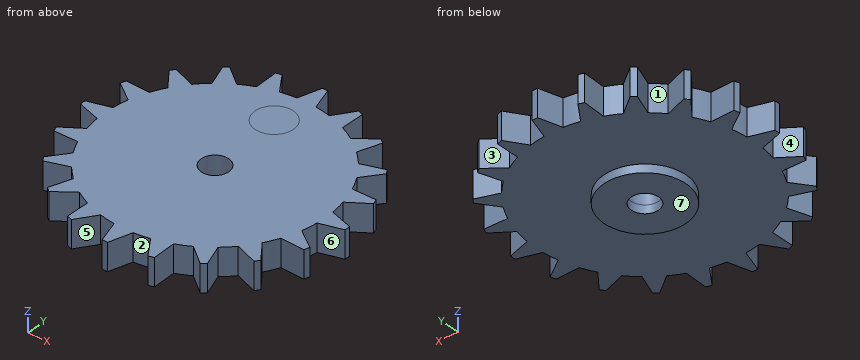
from build123d import *

# Parameters (mm, degrees)
SKETCH1_R           = 40
BOSS_EXTRUDE1_DEPTH = 10
SKETCH2_R           = 5
CUT_EXTRUDE1_DEPTH  = 10
BOSS_EXTRUDE2_DEPTH = 10
SKETCH4_R           = 5
BOSS_EXTRUDE3_DEPTH = 0.0001
SKETCH5_R           = 7
BOSS_EXTRUDE4_DEPTH = 0.0001
SKETCH6_R           = 15
BOSS_EXTRUDE5_DEPTH = 3
CUT_EXTRUDE2_START  = -3
SKETCH7_R           = 5
CUT_EXTRUDE2_DEPTH  = 3


with BuildPart() as part:
    # Sketch1 → Boss-Extrude1 (new body)
    with BuildSketch(Plane.XY):
        Circle(SKETCH1_R)
    extrude(amount=BOSS_EXTRUDE1_DEPTH)

    # Sketch2 → Cut-Extrude1 (cut)
    with BuildSketch(Plane.XY.offset(10)):
        Circle(SKETCH2_R)
    extrude(amount=-CUT_EXTRUDE1_DEPTH, mode=Mode.SUBTRACT)

    # Sketch3 → Boss-Extrude2 (add)
    with BuildSketch(Plane.XY.offset(10)):
        Polygon((-1, 48), (1, 48), (4, 38), (-4, 38), align=None)
        Polygon((7.938419721, 37.376215597), (13.881759214, 45.959729777), (15.783872246, 45.341695788), (15.546871851, 34.904079642), align=None)
        Polygon((19.09977161, 33.093786795), (27.404675116, 39.420600982), (29.022709104, 38.245030478), (25.571907565, 28.391504777), align=None)
        Polygon((28.391504777, 25.571907565), (38.245030478, 29.022709104), (39.420600982, 27.404675116), (33.093786795, 19.09977161), align=None)
        Polygon((34.904079642, 15.546871851), (45.341695788, 15.783872246), (45.959729777, 13.881759214), (37.376215597, 7.938419721), align=None)
        Polygon((38, 4), (48, 1), (48, -1), (38, -4), align=None)
        Polygon((37.376215597, -7.938419721), (45.959729777, -13.881759214), (45.341695788, -15.783872246), (34.904079642, -15.546871851), align=None)
        Polygon((33.093786795, -19.09977161), (39.420600982, -27.404675116), (38.245030478, -29.022709104), (28.391504777, -25.571907565), align=None)
        Polygon((25.571907565, -28.391504777), (29.022709104, -38.245030478), (27.404675116, -39.420600982), (19.09977161, -33.093786795), align=None)
        Polygon((15.546871851, -34.904079642), (15.783872246, -45.341695788), (13.881759214, -45.959729777), (7.938419721, -37.376215597), align=None)
        Polygon((4, -38), (1, -48), (-1, -48), (-4, -38), align=None)
        Polygon((-7.938419721, -37.376215597), (-13.881759214, -45.959729777), (-15.783872246, -45.341695788), (-15.546871851, -34.904079642), align=None)
        Polygon((-19.09977161, -33.093786795), (-27.404675116, -39.420600982), (-29.022709104, -38.245030478), (-25.571907565, -28.391504777), align=None)
        Polygon((-28.391504777, -25.571907565), (-38.245030478, -29.022709104), (-39.420600982, -27.404675116), (-33.093786795, -19.09977161), align=None)
        Polygon((-34.904079642, -15.546871851), (-45.341695788, -15.783872246), (-45.959729777, -13.881759214), (-37.376215597, -7.938419721), align=None)
        Polygon((-38, -4), (-48, -1), (-48, 1), (-38, 4), align=None)
        Polygon((-37.376215597, 7.938419721), (-45.959729777, 13.881759214), (-45.341695788, 15.783872246), (-34.904079642, 15.546871851), align=None)
        Polygon((-33.093786795, 19.09977161), (-39.420600982, 27.404675116), (-38.245030478, 29.022709104), (-28.391504777, 25.571907565), align=None)
        Polygon((-25.571907565, 28.391504777), (-29.022709104, 38.245030478), (-27.404675116, 39.420600982), (-19.09977161, 33.093786795), align=None)
        Polygon((-15.546871851, 34.904079642), (-15.783872246, 45.341695788), (-13.881759214, 45.959729777), (-7.938419721, 37.376215597), align=None)
    extrude(amount=-BOSS_EXTRUDE2_DEPTH)

    # Sketch4 → Boss-Extrude3 (add)
    with BuildSketch(Plane.XY.offset(10)):
        with Locations((-1.366858005, 27.473845905)):
            Circle(SKETCH4_R)
    extrude(amount=BOSS_EXTRUDE3_DEPTH)

    # Sketch5 → Boss-Extrude4 (add)
    with BuildSketch(Plane.XY.offset(10)):
        with Locations((-1.366858005, 27.473845905)):
            Circle(SKETCH5_R)
    extrude(amount=BOSS_EXTRUDE4_DEPTH)

    # Sketch6 → Boss-Extrude5 (add)
    with BuildSketch(Plane(origin=(0, 0, 0), x_dir=(-1, 0, 0), z_dir=(0, 0, -1))):
        with Locations(Location((0, 0, 0), (0, 0, 180))):
            Circle(SKETCH6_R)
    extrude(amount=BOSS_EXTRUDE5_DEPTH)

    # Sketch7 → Cut-Extrude2 (cut)
    with BuildSketch(Plane(origin=(0, 0, -3), x_dir=(-1, 0, 0), z_dir=(0, 0, -1)).offset(CUT_EXTRUDE2_START)):
        with Locations(Location((0, 0, 0), (0, 0, 180))):
            Circle(SKETCH7_R)
    extrude(amount=CUT_EXTRUDE2_DEPTH, mode=Mode.SUBTRACT)


solid = part.part
Source: CAD feature listing. Evaluate the final solid. Frame: model axes, mm. Face numbers are marked on the shaded views. A direction names the side the tool comes from. Round coordinates to 2 decimals unless told otherwise and drop trailing zeros. Order: outer loops, then holes, each group sorted by start corner. A loop starts at its lowest first (then second) coordinate and runs counter-clockwise, first axis right, second up. Notation, with made-up numbers: (38, -14) - (87, -14) arc R21 ccw to (87, -6) - close; hole circle Ø9 at (19, 53.5). An arc over 180 degrees is marked (long way). Use a Markdown table: item, result. Add a question column.
1. Section query A-A (y = -32). Return the cut outline in (x, z).
2. First-contact query: pin 1 (1 mm diameter, centred on y = 31.5, z = 8, fed in from -X); pin 2 (1 mm diameter, centred on x = -21.5, z = 8.5, fed in from +Y); pin 3 (6 mm diameter, centred on x = 32.5, y = 17.5, fed in from -Z); pin 4 (11.5 mm diameter, centred on x = 0, y = 0, fed in from -Z). Flat tips, straight axial feed; report the tip coordinate or a pass-through.
3. Set-up query: the marked faces 1, 2, 3 and 4. Return all of +Z, -Z, +X, -X, +Y, -Y with unobstructed straight access to the full face (end or side cutting, diameter ignored); none if empty.
4. Line query: probe 1 along Y at (x, z) = (0, -1.1); probe 2 along Y at (x, z) = (0, 3.75); probe 3 along X at (y, z) = (-37, 3.75). Output: solid intervals per line, ascending.
5. Mould query, pull axis X, two halves, no side actions, for the marked faces 5, 6 and 7. Classes: +X half, -X half, draft (parallel to the pull), parting line (faces both ways), or undercut.
Derived:
| question | item | result |
|---|---|---|
| 1 | outline | (-26.84, 0) - (26.84, 0) - (26.84, 10) - (-26.84, 10) - close |
| 2 | pin 1 | x = -26.84 |
| 2 | pin 2 | y = 35.3 |
| 2 | pin 3 | z = 0 |
| 2 | pin 4 | z = -3 |
| 3 | face 1 | +Z, -Z |
| 3 | face 2 | +Z, -Z, -Y |
| 3 | face 3 | +Z, -Z, +Y |
| 3 | face 4 | +Z, -Z, -X |
| 4 | probe 1 | -15 to -5, 5 to 15 |
| 4 | probe 2 | -48 to -5, 5 to 48 |
| 4 | probe 3 | -28.59 to -24.23, -15.59 to 15.59, 24.23 to 28.59 |
| 5 | face 5 | undercut |
| 5 | face 6 | +X half |
| 5 | face 7 | draft |
